Check sheet for the modelled part. Datum: model origin and axes. Units: mm. Round coordinates to 2 decimals unless told otherwise and drop trailing zeros. Write each loop counter-clockwise with the first axis right and the second up, starting at its lowest first coordinate (ties: lowest second). Pieces come first, ordered by that corner, then holes. Notation, with made-up numbers: M -7.75,-22 L 6.25,-22 A16 ccw 6.25,-10 Z; hole C 60.25,-35.75 d9. An arc over 180 degrees is marked long. Put each result on its own line as item: value.
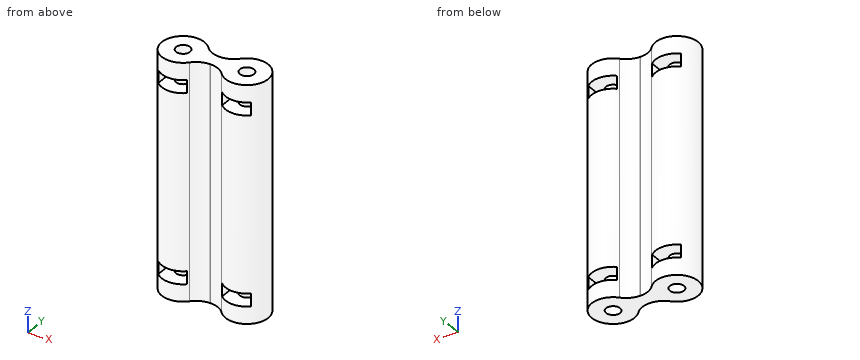
```python
from build123d import *

# Parameters (mm, degrees)
ESBO_O1_R                  = 1.65
RESSALTO_EXTRUS_O1_DEPTH   = 55
FILETE1_R                  = 5
CORTE_EXTRUS_O1_DEPTH      = 57.623758265
CORTE_EXTRUS_O1_DEPTH_BACK = 57.623758265
ESBO_O2_W                  = 6.8
ESBO_O2_H                  = 3


with BuildPart() as part:
    # Esboço1 → Ressalto-extrusão1 (new body)
    with BuildSketch(Plane.XY):
        with BuildLine():
            Line((-2.78009534, 1.65), (2.78009534, 1.65))
            ThreePointArc((2.78009534, 1.65), (12.5, 0), (2.78009534, -1.65))
            Line((2.78009534, -1.65), (-2.78009534, -1.65))
            ThreePointArc((-2.78009534, -1.65), (-12.5, 0), (-2.78009534, 1.65))
        make_face()
        with Locations((-7.5, 0)):
            Circle(ESBO_O1_R, mode=Mode.SUBTRACT)
        with Locations((7.5, 0)):
            Circle(ESBO_O1_R, mode=Mode.SUBTRACT)
    extrude(amount=RESSALTO_EXTRUS_O1_DEPTH)

    # Filete1
    filete1_edges = [part.edges().sort_by_distance(p)[0] for p in [
        (-2.78009534, 1.65, 27.5),
        (2.78009534, 1.65, 27.5),
        (2.78009534, -1.65, 27.5),
        (-2.78009534, -1.65, 27.5),
    ]]
    fillet(filete1_edges, radius=FILETE1_R)

    # Esboço2 → Corte-extrusão1 (cut, two sides: drawn at the far end of the back side and taken through both)
    with BuildSketch(Plane(origin=(0, 0, 0), x_dir=(1, 0, 0), z_dir=(0, 1, 0)).offset(-CORTE_EXTRUS_O1_DEPTH_BACK)):
        with Locations((-7.5, -5.5)):
            Rectangle(ESBO_O2_W, ESBO_O2_H)
        with Locations((7.5, -5.5)):
            Rectangle(ESBO_O2_W, ESBO_O2_H)
        with Locations((7.5, -49.5)):
            Rectangle(ESBO_O2_W, ESBO_O2_H)
        with Locations((-7.5, -49.5)):
            Rectangle(ESBO_O2_W, ESBO_O2_H)
    extrude(amount=CORTE_EXTRUS_O1_DEPTH + CORTE_EXTRUS_O1_DEPTH_BACK, mode=Mode.SUBTRACT)


solid = part.part
```
1. Scan lines: probe 1 along Z at (x, y) = (-4.5, 2.5); probe 2 along X at (y, z) = (0, 36.5); probe 3 along Y at (x, z) = (7.5, 26). Record each from-to range of solid material in increasing order.
Computed values:
probe 1: z = 0 to 4, 7 to 48, 51 to 55
probe 2: x = -12.5 to -9.15, -5.85 to 5.85, 9.15 to 12.5
probe 3: y = -5 to -1.65, 1.65 to 5
2. Cross-section at A-A (z = 5.5). Enter the section's corners in (x, y) (3 decimals).
Computed values:
outline: M -10.9,-3.666 L -10.9,3.666 A5 ccw Z; M -4.1,-3.666 A5 ccw -3.766,-3.325 A5 cw -0.032,-1.65 L 0.032,-1.65 A5 cw 3.766,-3.325 A5 ccw 4.1,-3.666 L 4.1,3.666 A5 ccw 3.766,3.325 A5 cw 0.032,1.65 L -0.032,1.65 A5 cw -3.766,3.325 A5 ccw -4.1,3.666 Z; M 10.9,-3.666 A5 ccw 10.9,3.666 Z
3. Cross-section at D-D (y = 0). Count the separate pieces of the cut face and the enclosed holes in it, then the cut area to 3 significant figures.
Computed values:
separate pieces: 3
enclosed holes: 0
area: 970 mm2
4. Cross-section at C-C (x = -7.5). Enter the section's corners in (y, z), then the cut area to 3 significant figures.
Computed values:
outline: M -5,0 L -1.65,0 L -1.65,4 L -5,4 Z; M -5,7 L -1.65,7 L -1.65,48 L -5,48 Z; M -5,51 L -1.65,51 L -1.65,55 L -5,55 Z; M 1.65,0 L 5,0 L 5,4 L 1.65,4 Z; M 1.65,7 L 5,7 L 5,48 L 1.65,48 Z; M 1.65,51 L 5,51 L 5,55 L 1.65,55 Z
area: 328 mm2
5. Depth check by flat-ended pin: pin 1 Ø1.5 at (y, z) = (4, 25.5) entering from -X; pin 2 Ø2.5 at (y, z) = (-1.5, 50) entering from +X. Enter the tip coordinate at first touch or a pass-through.
Computed values:
pin 1: stops at x = -11.3
pin 2: stops at x = 12.49
6. Cross-section at B-B (y = -2.5). Enter the section's corners in (x, z), then the cut area to 3 significant figures.
Computed values:
outline: M -11.83,0 L -2.82,0 L -2.82,55 L -11.83,55 Z; M 2.82,0 L 11.83,0 L 11.83,55 L 2.82,55 Z; hole M -10.9,4 L -4.1,4 L -4.1,7 L -10.9,7 Z; hole M -10.9,48 L -4.1,48 L -4.1,51 L -10.9,51 Z; hole M 4.1,4 L 10.9,4 L 10.9,7 L 4.1,7 Z; hole M 4.1,48 L 10.9,48 L 10.9,51 L 4.1,51 Z
area: 909 mm2
